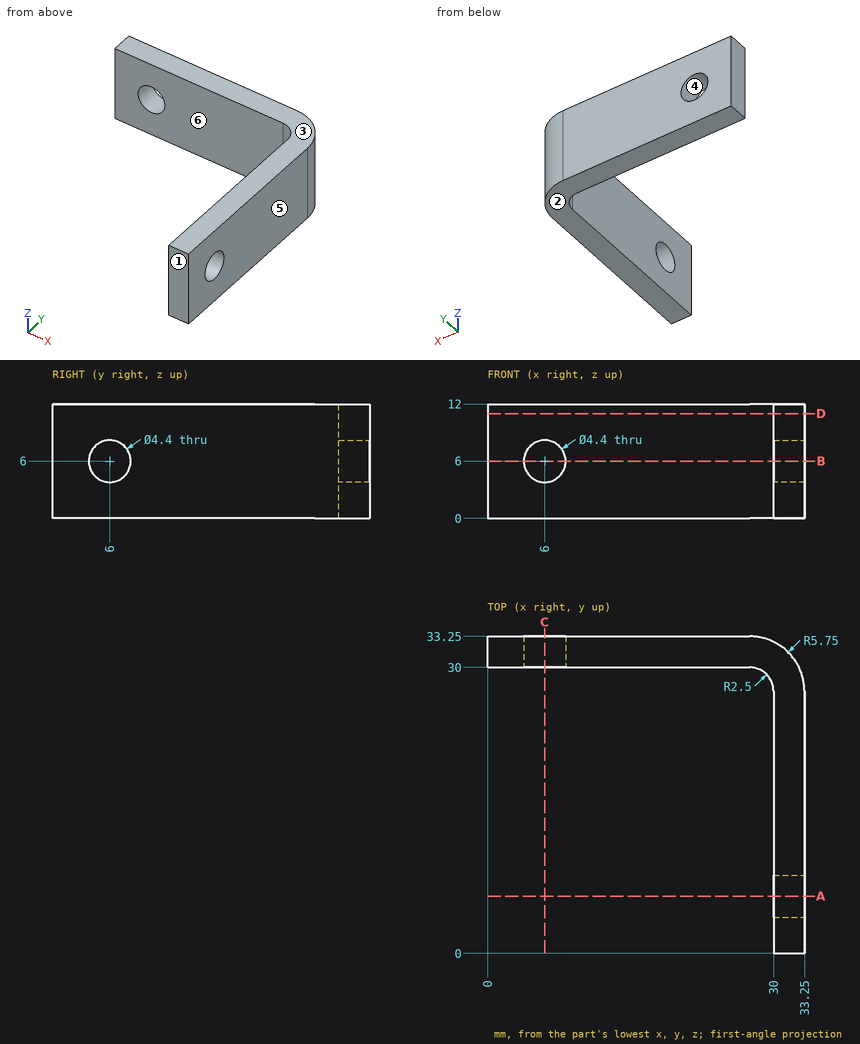
Input: dimensioned drawing with shaded views. Units: mm. Origin: part minimum x, y, z. A direction names the side the tool comes from. Give positions to 0.01 mm unless a question says otherwise; leave off trailing zeros. Order: outer loops, then holes, each group sorted by start corner. A loop starts at its lowest first (then second) coordinate and runs counter-clockwise, first axis right, second up. Notation, with made-up numbers: (35, 77) -> (64, 77) arc R7 ccw to (64, 87) -> close; hole circle Ø4 at (46.5, 47.25). An arc over 180 degrees is marked (long way). Use one line per item in the form item = value.
1) Mould query, pull axis Z, two halves, no side actions, for the marked faces 1, 2, 3 and 4. Classes: pulls with the +Z half, pulls with the -Z half, needs draft (parallel to the pull), parting line crosses it, or undercut.
Response values:
face_1 = needs draft
face_2 = pulls with the -Z half
face_3 = pulls with the +Z half
face_4 = undercut
2) Line query: probe 1 along Z at (x, y) = (6, 31); probe 2 along X at (y, z) = (6, 8.75). Output: solid intervals per line, ascending.
Response values:
probe_1 = 0 to 3.8, 8.2 to 12
probe_2 = 30 to 33.25
3) Reachability of the marked faces 5 and 6 from +Z, -Z, +X, -X, +Y, -Y: full face, straight path, thin tool, end or side. Return the list, or none.
Response values:
face_5 = +Z, -Z, +X, +Y, -Y
face_6 = +Z, -Z, -X, -Y
4) Section A-A, the plane y = 6. Return loops of the section in (x, z).
Response values:
outline = (30, 0) -> (33.25, 0) -> (33.25, 3.8) -> (30, 3.8) -> close; (30, 8.2) -> (33.25, 8.2) -> (33.25, 12) -> (30, 12) -> close
5) Section B-B, the plane z = 6. Return loops of the section in (x, y).
Response values:
outline = (0, 30) -> (3.8, 30) -> (3.8, 33.25) -> (0, 33.25) -> close; (8.2, 30) -> (27.5, 30) arc R2.5 cw to (30, 27.5) -> (30, 8.2) -> (33.25, 8.2) -> (33.25, 27.5) arc R5.75 ccw to (27.5, 33.25) -> (8.2, 33.25) -> close; (30, 0) -> (33.25, 0) -> (33.25, 3.8) -> (30, 3.8) -> close
6) Section D-D, the plane z = 11. Return loops of the section in (x, y).
Response values:
outline = (0, 30) -> (27.5, 30) arc R2.5 cw to (30, 27.5) -> (30, 0) -> (33.25, 0) -> (33.25, 27.5) arc R5.75 ccw to (27.5, 33.25) -> (0, 33.25) -> close
7) First-contact query: pin 1 Ø5 at (x, z) = (6, 6) entering from +Y; pin 2 Ø3.5 at (y, z) = (11, 5.5) entering from -X; pin 3 Ø1 at (y, z) = (27.5, 9.5) entering from -X. Flat tips, straight axial feed; report the tip coordinate or a pass-through.
Response values:
pin_1 = 33.25
pin_2 = 30
pin_3 = 29.95
